Part model, mm, in its own coordinate system. Give positions to 0.01 mm unless a question says otherwise; leave off trailing zeros. Order: outer loops, then holes, each group sorted by start corner. A loop starts at its lowest first (then second) coordinate and runs counter-clockwise, first axis right, second up. Notation, with made-up numbers: (77, 34) -> (95, 34) arc R28 ccw to (95, 62) -> close; hole circle Ø8 at (3, -2.5). An arc over 180 degrees is marked (long way). Write item = value, one per line. Start each with the question number.
(1) Probe line 1 along Z through (x, y) = (76.2, 3); line 2 along X through (y, z) = (4, -63.5); line 3 along Z through (x, y) = (49.5, 3.25). List the from-to ranges inside material, lowest first. Write a range as from..to.
(2) Saw through at C-C, the plane z = -38.1. State how many separate pieces and enclosed holes the cut face has, then the cut area to 3 significant figures.
(3) Saw through at D-D, the plane x = 76.2. List the corners of the cut face in (y, z), then the cut area to 3 significant figures.
(4) Flat gauge pins, fed straight in: pin 1 (3 mm diameter, centred on y = 3, z = -74.5, fed in from -X); pin 2 (4 mm diameter, centred on x = 88.9, z = -127, fed in from -Y); pin 3 (2 mm diameter, centred on x = 26.5, y = 3, fed in from -Z); pin 4 (1 mm diameter, centred on x = 53, y = 3, fed in from -Z). Where does each tip first touch, or does it go through?
(5) Saw through at B-B, the plane x = 38.1. List the corners of the cut face in (y, z).
(6) Saw through at A-A, the plane z = -139.7. List the corners of the cut face in (x, y), then the cut area to 3 significant figures.
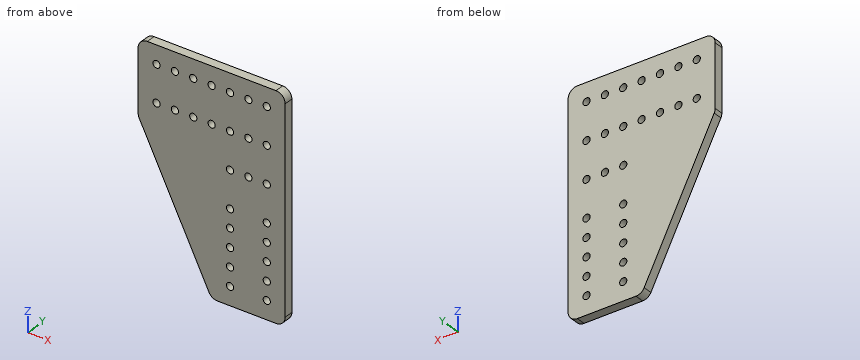
from build123d import *

# Parameters (mm, degrees)
BOSS_EXTRUDE1_DEPTH = 6.35
SKETCH2_R           = 2.4892
CUT_EXTRUDE1_DEPTH  = 7.35
FILLET1_R           = 6.35


with BuildPart() as part:
    # Sketch1 → Boss-Extrude1 (new body)
    with BuildSketch(Plane(origin=(0, 0, 0), x_dir=(1, 0, 0), z_dir=(0, 1, 0))):
        Polygon((0, 50.8), (50.8, 152.4), (101.6, 152.4), (101.6, 0), (0, 0), align=None)
    extrude(amount=BOSS_EXTRUDE1_DEPTH)

    # Sketch2 → Cut-Extrude1 (cut, through all)
    with BuildSketch(Plane(origin=(0, 6.35, 0), x_dir=(1, 0, 0), z_dir=(0, 1, 0))):
        with Locations((88.9, 12.7)):
            Circle(SKETCH2_R)
        with Locations((76.2, 12.7)):
            Circle(SKETCH2_R)
        with Locations((63.5, 12.7)):
            Circle(SKETCH2_R)
        with Locations((50.8, 12.7)):
            Circle(SKETCH2_R)
        with Locations((38.1, 12.7)):
            Circle(SKETCH2_R)
        with Locations((25.4, 12.7)):
            Circle(SKETCH2_R)
        with Locations((12.7, 12.7)):
            Circle(SKETCH2_R)
        with Locations((76.2, 38.1)):
            Circle(SKETCH2_R)
        with Locations((63.5, 38.1)):
            Circle(SKETCH2_R)
        with Locations((50.8, 38.1)):
            Circle(SKETCH2_R)
        with Locations((38.1, 38.1)):
            Circle(SKETCH2_R)
        with Locations((25.4, 38.1)):
            Circle(SKETCH2_R)
        with Locations((12.7, 38.1)):
            Circle(SKETCH2_R)
        with Locations((76.2, 63.5)):
            Circle(SKETCH2_R)
        with Locations((63.5, 63.5)):
            Circle(SKETCH2_R)
        with Locations((63.5, 88.9)):
            Circle(SKETCH2_R)
        with Locations((63.5, 101.6)):
            Circle(SKETCH2_R)
        with Locations((63.5, 114.3)):
            Circle(SKETCH2_R)
        with Locations((63.5, 127)):
            Circle(SKETCH2_R)
        with Locations((63.5, 139.7)):
            Circle(SKETCH2_R)
        with Locations((88.9, 38.1)):
            Circle(SKETCH2_R)
        with Locations((88.9, 63.5)):
            Circle(SKETCH2_R)
        with Locations((88.9, 88.9)):
            Circle(SKETCH2_R)
        with Locations((88.9, 101.6)):
            Circle(SKETCH2_R)
        with Locations((88.9, 114.3)):
            Circle(SKETCH2_R)
        with Locations((88.9, 127)):
            Circle(SKETCH2_R)
        with Locations((88.9, 139.7)):
            Circle(SKETCH2_R)
    extrude(amount=-CUT_EXTRUDE1_DEPTH, mode=Mode.SUBTRACT)

    # Fillet1
    fillet1_edges = [part.edges().sort_by_distance(p)[0] for p in [
        (0, 3.175, -50.8),
        (50.8, 3.175, -152.4),
        (101.6, 3.175, -152.4),
        (101.6, 3.175, 0),
        (0, 3.175, 0),
    ]]
    fillet(fillet1_edges, radius=FILLET1_R)


solid = part.part
Results list:
q1.line_1 = -152.4..-65.99, -61.01..-40.59, -35.61..-15.19, -10.21..0
q1.line_2 = 6.35..61.01, 65.99..73.71, 78.69..86.41, 91.39..101.6
q1.line_3 = -149.66..-40.22, -35.98..-14.82, -10.58..0
q2.separate_pieces = 8
q2.enclosed_holes = 0
q2.area = 424 mm^2
q3.outline = (0, -152.4) -> (6.35, -152.4) -> (6.35, -65.99) -> (0, -65.99) -> close; (0, -61.01) -> (6.35, -61.01) -> (6.35, -40.59) -> (0, -40.59) -> close; (0, -35.61) -> (6.35, -35.61) -> (6.35, -15.19) -> (0, -15.19) -> close; (0, -10.21) -> (6.35, -10.21) -> (6.35, 0) -> (0, 0) -> close
q3.area = 873 mm^2
q4.pin_1 = 11.1
q4.pin_2 = through
q4.pin_3 = -105.8
q4.pin_4 = -152.28
q5.outline = (0, -127) -> (6.35, -127) -> (6.35, -40.59) -> (0, -40.59) -> close; (0, -35.61) -> (6.35, -35.61) -> (6.35, -15.19) -> (0, -15.19) -> close; (0, -10.21) -> (6.35, -10.21) -> (6.35, 0) -> (0, 0) -> close
q6.outline = (44.45, 0) -> (61.01, 0) -> (61.01, 6.35) -> (44.45, 6.35) -> close; (65.99, 0) -> (86.41, 0) -> (86.41, 6.35) -> (65.99, 6.35) -> close; (91.39, 0) -> (101.6, 0) -> (101.6, 6.35) -> (91.39, 6.35) -> close
q6.area = 300 mm^2
